Source: CAD feature listing. Evaluate the final solid. Frame: model axes, mm. A direction names the side the tool comes from. Coordinates: 2 decimals unless noted, no trailing zeros. Order: outer loops, then holes, each group sorted by start corner. A loop starts at its lowest first (then second) coordinate and runs counter-clockwise, first axis right, second up.
```python
from build123d import *

# Parameters (mm, degrees)
EXTRUDE_1_DEPTH     = 43
EXTRUDE_2_DEPTH     = 8.6
SKETCH_3_R          = 1.4
CUT_EXTRUDE_1_DEPTH = 15
CUT_EXTRUDE_START   = -17.2
SKETCH_4_R          = 2.5
CUT_EXTRUDE_2_DEPTH = 17.2
SKETCH_5_W          = 5
SKETCH_5_H          = 10
CUT_EXTRUDE_3_DEPTH = 15
SKETCH_6_R          = 1.7
CUT_EXTRUDE_4_DEPTH = 20
CUT_EXTRUDE_START_2 = -3
SKETCH_7_W          = 2.192810324
SKETCH_7_H          = 3
SKETCH_7_R          = 1.7
CUT_EXTRUDE_5_DEPTH = 3
FILLET_1_R          = 3
FILLET_2_R          = 1


with BuildPart() as part:
    # Эскиз1 → Бобышка-Вытянуть1 (new body)
    with BuildSketch(Plane.XY):
        with BuildLine():
            Line((5.85, 0), (5.85, 11.699503018))
            ThreePointArc((5.85, 11.699503018), (0, 14.42), (-5.85, 11.699503018))
            Line((-5.85, 11.699503018), (-5.85, 0))
            Line((-5.85, 0), (-12.85, 0))
            Line((-12.85, 0), (-12.85, 17.2))
            Line((-12.85, 17.2), (12.85, 17.2))
            Line((12.85, 17.2), (12.85, 0))
            Line((12.85, 0), (5.85, 0))
        make_face()
    extrude(amount=EXTRUDE_1_DEPTH)

    # Эскиз2 → Бобышка-Вытянуть2 (add)
    with BuildSketch(Plane(origin=(0, 17.2, 0), x_dir=(1, 0, 0), z_dir=(0, 1, 0))):
        with BuildLine():
            Line((-12.85, -7.5), (-8.85, -7.5))
            ThreePointArc((-8.85, -7.5), (-6.728679656, -8.378679656), (-5.85, -10.5))
            Line((-5.85, -10.5), (-5.85, -32.5))
            ThreePointArc((-5.85, -32.5), (-6.728679656, -34.621320344), (-8.85, -35.5))
            Line((-8.85, -35.5), (-12.85, -35.5))
            Line((-12.85, -35.5), (-12.85, -24))
            ThreePointArc((-12.85, -24), (-10.35, -21.5), (-12.85, -19))
            Line((-12.85, -19), (-12.85, -7.5))
        make_face()
    extrude(amount=EXTRUDE_2_DEPTH)

    # Эскиз3 → Вырез-Вытянуть1 (cut)
    with BuildSketch(Plane(origin=(0, 25.8, 0), x_dir=(1, 0, 0), z_dir=(0, 1, 0))):
        with Locations(Location((-10.35, -10.5, 0), (0, 0, 270))):
            Circle(SKETCH_3_R)
        with Locations(Location((-10.35, -32.5, 0), (0, 0, 90))):
            Circle(SKETCH_3_R)
    extrude(amount=-CUT_EXTRUDE_1_DEPTH, mode=Mode.SUBTRACT)

    # Эскиз4 → Вырез-Вытянуть2 (cut)
    with BuildSketch(Plane(origin=(0, 17.2, 0), x_dir=(1, 0, 0), z_dir=(0, 1, 0)).offset(CUT_EXTRUDE_START)):
        with Locations((-12.85, -21.5)):
            Circle(SKETCH_4_R)
    extrude(amount=CUT_EXTRUDE_2_DEPTH, mode=Mode.SUBTRACT)

    # Эскиз5 → Вырез-Вытянуть3 (cut)
    with BuildSketch(Plane.ZY.offset(12.85)):
        with Locations((21.5, 5)):
            Rectangle(SKETCH_5_W, SKETCH_5_H)
    extrude(amount=-CUT_EXTRUDE_3_DEPTH, mode=Mode.SUBTRACT)

    # Эскиз6 → Вырез-Вытянуть4 (cut)
    with BuildSketch(Plane.XZ):
        with Locations((9.5, 39)):
            Circle(SKETCH_6_R)
        with Locations(Location((-9.5, 39, 0), (0, 0, 270))):
            Circle(SKETCH_6_R)
        with Locations(Location((9.5, 4, 0), (0, 0, 270))):
            Circle(SKETCH_6_R)
        with Locations((-9.5, 4)):
            Circle(SKETCH_6_R)
    extrude(amount=-CUT_EXTRUDE_4_DEPTH, mode=Mode.SUBTRACT)

    # Эскиз7 → Вырез-Вытянуть5 (cut)
    # profile 1 of 8: a face of its own
    with BuildSketch(Plane(origin=(0, 17.2, 0), x_dir=(1, 0, 0), z_dir=(0, 1, 0)).offset(CUT_EXTRUDE_START_2)):
        with Locations((-13.946405162, -4)):
            Rectangle(SKETCH_7_W, SKETCH_7_H)
    # profile 2 of 8: a face of its own
    with BuildSketch(Plane(origin=(0, 17.2, 0), x_dir=(1, 0, 0), z_dir=(0, 1, 0)).offset(CUT_EXTRUDE_START_2)):
        Polygon((-12.85, -5.5), (-11.867136104, -5.5), (-11.116580754, -6.8), (-7.883419246, -6.8), (-6.266838493, -4), (-7.883419246, -1.2), (-11.116580754, -1.2), (-11.867136104, -2.5), (-12.85, -2.5), align=None)
        with Locations((-9.5, -4)):
            Circle(SKETCH_7_R, mode=Mode.SUBTRACT)
    # profile 3 of 8: a face of its own
    with BuildSketch(Plane(origin=(0, 17.2, 0), x_dir=(1, 0, 0), z_dir=(0, 1, 0)).offset(CUT_EXTRUDE_START_2)):
        Polygon((12.85, -5.5), (12.85, -2.5), (11.867136104, -2.5), (11.116580754, -1.2), (7.883419246, -1.2), (6.266838493, -4), (7.883419246, -6.8), (11.116580754, -6.8), (11.867136104, -5.5), align=None)
        with Locations(Location((9.5, -4, 0), (0, 0, 270))):
            Circle(SKETCH_7_R, mode=Mode.SUBTRACT)
    # profile 4 of 8: a face of its own
    with BuildSketch(Plane(origin=(0, 17.2, 0), x_dir=(1, 0, 0), z_dir=(0, 1, 0)).offset(CUT_EXTRUDE_START_2)):
        with Locations((13.946405162, -4)):
            Rectangle(SKETCH_7_W, SKETCH_7_H)
    # profile 5 of 8: a face of its own
    with BuildSketch(Plane(origin=(0, 17.2, 0), x_dir=(1, 0, 0), z_dir=(0, 1, 0)).offset(CUT_EXTRUDE_START_2)):
        with Locations((13.946405162, -39)):
            Rectangle(SKETCH_7_W, SKETCH_7_H)
    # profile 6 of 8: a face of its own
    with BuildSketch(Plane(origin=(0, 17.2, 0), x_dir=(1, 0, 0), z_dir=(0, 1, 0)).offset(CUT_EXTRUDE_START_2)):
        Polygon((12.85, -40.5), (12.85, -37.5), (11.867136104, -37.5), (11.116580754, -36.2), (7.883419246, -36.2), (6.266838493, -39), (7.883419246, -41.8), (11.116580754, -41.8), (11.867136104, -40.5), align=None)
        with Locations((9.5, -39)):
            Circle(SKETCH_7_R, mode=Mode.SUBTRACT)
    # profile 7 of 8: a face of its own
    with BuildSketch(Plane(origin=(0, 17.2, 0), x_dir=(1, 0, 0), z_dir=(0, 1, 0)).offset(CUT_EXTRUDE_START_2)):
        Polygon((-11.867136104, -37.5), (-12.85, -37.5), (-12.85, -40.5), (-11.867136104, -40.5), (-11.116580754, -41.8), (-7.883419246, -41.8), (-6.266838493, -39), (-7.883419246, -36.2), (-11.116580754, -36.2), align=None)
        with Locations(Location((-9.5, -39, 0), (0, 0, 270))):
            Circle(SKETCH_7_R, mode=Mode.SUBTRACT)
    # profile 8 of 8: a face of its own
    with BuildSketch(Plane(origin=(0, 17.2, 0), x_dir=(1, 0, 0), z_dir=(0, 1, 0)).offset(CUT_EXTRUDE_START_2)):
        with Locations((-13.946405162, -39)):
            Rectangle(SKETCH_7_W, SKETCH_7_H)
    extrude(amount=CUT_EXTRUDE_5_DEPTH, mode=Mode.SUBTRACT)

    # Скругление1
    fillet_1_edges = [part.edges().sort_by_distance(p)[0] for p in [
        (-5.85, 5, 24),
        (-5.85, 5, 19),
    ]]
    fillet(fillet_1_edges, radius=FILLET_1_R)

    # Скругление2
    fillet_2_edges = [part.edges().sort_by_distance(p)[0] for p in [
        (12.85, 8.6, 0),
        (-12.85, 8.6, 0),
        (12.85, 8.6, 43),
        (-12.85, 8.6, 43),
        (-12.85, 21.5, 35.5),
        (-12.85, 21.5, 7.5),
    ]]
    fillet(fillet_2_edges, radius=FILLET_2_R)


solid = part.part
```
1. Draft query along Z for faces 1 (the face through (-12.549, 21.56, 35.215)), 2 (the face through (-12.549, 21.56, 7.785)), 3 (the face through (-12.85, 10, 10)), 4 (the face through (-9, 16, 1.2)). Return one class per face: released by +Z, released by -Z, zero draft, split by the parting line, or undercut.
Findings:
face 1: released by +Z
face 2: released by -Z
face 3: zero draft
face 4: undercut
2. Section query B-B on x = 9.5. Return loops of the section in (y, z), plus the area to 3 significant figures.
Findings:
outline: (0, 0) - (17.2, 0) - (17.2, 1.2) - (14.2, 1.2) - (14.2, 2.3) - (0, 2.3) - close; (0, 5.7) - (14.2, 5.7) - (14.2, 6.8) - (17.2, 6.8) - (17.2, 36.2) - (14.2, 36.2) - (14.2, 37.3) - (0, 37.3) - close; (0, 40.7) - (14.2, 40.7) - (14.2, 41.8) - (17.2, 41.8) - (17.2, 43) - (0, 43) - close
area: 609 mm2
3. Ray query, line 1 (Z direction, x = 9.5, y = 10); line 2 (X direction, y = 10.25, z = 4); line 3 (X direction, y = 9.5, z = 36.5). Return the intervals inside material, ascending.
Findings:
line 1: z = 0 to 2.3, 5.7 to 37.3, 40.7 to 43
line 2: x = -12.85 to -11.2, -7.8 to -5.85, 5.85 to 7.8, 11.2 to 12.85
line 3: x = -12.85 to -5.85, 5.85 to 12.85
4. Pin query (flat end, axial travel): P1, Ø5, axis at x = -4, y = 21.5, coming from the +Z side; P2, Ø4, axis at x = -3, z = 21.5, coming from the +Y side; P3, Ø2.5, axis at x = -9.5, z = 39, coming from the +Y side; P4, Ø0.8, axis at x = -12.5, y = 15, coming from the -Z side. Return the tip coordinate at first contact, or that it passes through.
Findings:
P1: stops at z = 34.36
P2: stops at y = 17.2
P3: passes through
P4: stops at z = 0.03
5. Section query D-D on z = 27.5. Return loops of the section in (x, y), plus the area to 3 significant figures.
Findings:
outline: (-12.85, 0) - (-5.85, 0) - (-5.85, 11.7) arc R7.65 cw to (5.85, 11.7) - (5.85, 0) - (12.85, 0) - (12.85, 17.2) - (-5.85, 17.2) - (-5.85, 25.8) - (-12.85, 25.8) - close
area: 343 mm2
6. Access query for faces 5 (the face through (-10, 21, 7.5)), 6 (the face through (-11, 5, 19)), 7 (the face through (-11.487, 15.679, 1.841)), 8 (the face through (12.4, 15.7, 37.5)), 9 (the face through (-12.4, 15.7, 40.5)). Directions: +Z, -Z, +X, -X, +Y, -Y. A direction counts if a zero-diameter tool reaches every point of the face in a straight line with its end or side. Return the directions, or none.
Findings:
face 5: -Z, +X, -X, +Y
face 6: -X, -Y
face 7: +Y
face 8: +X, +Y
face 9: -X, +Y
7. Section query C-C on y = 21.5. Return loops of the section in (x, z), plus the area to 3 significant figures.
Findings:
outline: (-12.85, 8.5) arc R1 ccw to (-11.85, 7.5) - (-8.85, 7.5) arc R3 ccw to (-5.85, 10.5) - (-5.85, 32.5) arc R3 ccw to (-8.85, 35.5) - (-11.85, 35.5) arc R1 ccw to (-12.85, 34.5) - (-12.85, 24) arc R2.5 cw to (-12.85, 19) - close; hole circle Ø2.8 at (-10.35, 10.5); hole circle Ø2.8 at (-10.35, 32.5)
area: 170 mm2
8. Section query A-A on y = 7.5. Return loops of the section in (x, z).
Findings:
outline: (-12.85, 1) arc R1 ccw to (-11.85, 0) - (-5.85, 0) - (-5.85, 16) arc R3 ccw to (-8.85, 19) - (-12.85, 19) - close; (-12.85, 24) - (-8.85, 24) arc R3 ccw to (-5.85, 27) - (-5.85, 43) - (-11.85, 43) arc R1 ccw to (-12.85, 42) - close; (5.85, 0) - (11.85, 0) arc R1 ccw to (12.85, 1) - (12.85, 42) arc R1 ccw to (11.85, 43) - (5.85, 43) - close; hole circle Ø3.4 at (-9.5, 4); hole circle Ø3.4 at (-9.5, 39); hole circle Ø3.4 at (9.5, 4); hole circle Ø3.4 at (9.5, 39)
